from build123d import *

# Parameters (mm, degrees)
F0_W     = 99.999961
F0_H     = 100
F1_DEPTH = 100
F2_R     = 10.792816
F3_DEPTH = 50
F5_R     = 10.230309
F6_DEPTH = 50
F8_D     = 50


with BuildPart() as f1:
    # F0 (on Front) → F1 (new body)
    with BuildSketch(Plane.XZ):
        with Locations((49.99998, 50)):
            Rectangle(F0_W, F0_H)
    extrude(amount=F1_DEPTH)

    # F2 (on face) → F3 (join)
    with BuildSketch(Plane.XY.offset(100)):
        with Locations((48.785694, -51.932942)):
            Circle(F2_R)
    extrude(amount=F3_DEPTH)

    # F5 (on face) → F6 (join)
    with BuildSketch(Plane(origin=(0, 0, 0), x_dir=(1, 0, 0), z_dir=(0, 0, -1))):
        with Locations((50.976809, 52.556667)):
            Circle(F5_R)
    extrude(amount=F6_DEPTH)

    # F8 (through all)
    with Locations(Plane.YZ.offset(99.999961)):
        with Locations((-61.129767, 50.035987)):
            Hole(F8_D / 2)


solid = f1.part
Read the model definition and answer for the solid it produces. Units are mm, in the model's axes. A direction names the side the tool comes from. Give positions to 0.01 mm unless a question says otherwise; leave off trailing zeros. Loops run counter-clockwise (first coordinate to the right, second up) from the corner with the lowest first, then second, coordinate; pieces in that order, holes last. Notation, with made-up numbers: (24.25, 83.5) -> (78.25, 83.5) arc R17 ccw to (78.25, 89.5) -> close; hole circle Ø11 at (80.25, 30). An arc over 180 degrees is marked (long way). Answer as CSV lines item,"result".
Item 1: Find section D-D on y = -58. Give the vertices of the cut face in (x, z), plus the area to 3 significant figures.
Returned:
outline,"(0, 0) -> (42.31, 0) -> (42.31, -50) -> (59.64, -50) -> (59.64, 0) -> (100, 0) -> (100, 25.23) -> (0, 25.23) -> close; (0, 74.84) -> (100, 74.84) -> (100, 100) -> (57.71, 100) -> (57.71, 150) -> (39.86, 150) -> (39.86, 100) -> (0, 100) -> close"
area,"6,800 mm²"
Item 2: Consider line 1 (Y direction, x = 80.5, z = 49.5); line 2 (Z direction, x = 7, y = -32); line 3 (Z direction, x = 84, y = -76.5). Determine where each line is inside the solid, lowest interval first. Write a range as [from, to].
Returned:
line 1,"y = [-100, -86.12], [-36.14, 0]"
line 2,"z = [0, 100]"
line 3,"z = [0, 30.32], [69.75, 100]"
Item 3: Find section C-C on x = 54. Give the vertices of the cut face in (y, z), plus the area to 3 significant figures.
Returned:
outline,"(-100, 0) -> (-62.33, 0) -> (-62.33, -50) -> (-42.78, -50) -> (-42.78, 0) -> (0, 0) -> (0, 100) -> (-42.48, 100) -> (-42.48, 150) -> (-61.38, 150) -> (-61.38, 100) -> (-100, 100) -> close; hole circle Ø50 at (-61.13, 50.04)"
area,"9,960 mm²"
Item 4: Find section A-A on z = 58. Give the vertices of the cut face in (x, y).
Returned:
outline,"(0, -100) -> (100, -100) -> (100, -84.83) -> (0, -84.83) -> close; (0, -37.43) -> (100, -37.43) -> (100, 0) -> (0, 0) -> close"
Item 5: Each of these flat-tipped pins is pushed along its axis until it touches: pin 1 (3 mm diameter, centred on x = 35, y = -23, fed in from +Z); pin 2 (3 mm diameter, centred on x = 23, y = -61.5, fed in from -Z); pin 3 (4 mm diameter, centred on x = 47.5, z = -5.5, fed in from +Y). Where does it stop, or does it pass through?
Returned:
pin 1,"stops at z = 100"
pin 2,"stops at z = 0"
pin 3,"stops at y = -42.43"
Item 6: Determine the mould class of faces 3 (the face through (43.437, -59.471, -24.65)), 4 (the face through (0, -38, 38)), 5 (the face through (49.3, -74.57, 71.116)) for opening direction Y: +Y half, -Y half, draft (parallel to the pull), parting line (faces both ways), or undercut.
Returned:
face 3,"parting line"
face 4,"draft"
face 5,"undercut"
Item 7: Find section B-B on y = -39. Give the vertices of the cut face in (x, z).
Returned:
outline,"(0, 0) -> (100, 0) -> (100, 38.41) -> (0, 38.41) -> close; (0, 61.67) -> (100, 61.67) -> (100, 100) -> (0, 100) -> close"
Item 8: For faces 1 (the face through (49, -52, 150)), 2 (the face through (38, -51.5, 124.6)), determine the directions among +Z, -Z, +X, -X, +Y, -Y from which every point of the face is accessible in a straight line to the end or side of a thin tool.
Returned:
face 1,"+Z, +X, -X, +Y, -Y"
face 2,"+Z"
